Here's how the part is built. I have some questions about the finished solid (model axes, mm). Face numbers are marked on the shaded views. Give positions to 0.01 mm unless a question says otherwise; leave off trailing zeros. Write each loop counter-clockwise with the first axis right and the second up, starting at its lowest first coordinate (ties: lowest second). Pieces come first, ordered by that corner, then holes. Notation, with made-up numbers: (8, 14) - (14, 14) arc R20 cw to (14, 43) - close; hole circle Ø9 at (-6, -35.5). An arc over 180 degrees is marked (long way). One line per item, written item: value. Start each with the question number.
1) I'm going to push flat-ended pins straight in: P1, Ø3.5, axis at x = -12, z = 13, coming from the -Y side; P2, Ø0.9, axis at y = 1.5, z = 2, coming from the +X side; P3, Ø4.5, axis at y = -2, z = 22.5, coming from the -X side; P4, Ø3.5, axis at x = 35.24, y = 12.83, coming from the -Z side. Where does each tip first touch, or does it pass through?
2) Imagine slicing it at A-A on x = 0. Write out the boundary of the cut face in (y, z), plus the area to 3 significant figures.
3) Imagine slicing it at D-D on y = -24. Write out the boundary of the cut face in (x, z).
4) Imagine slicing it at B-B on y = 0. Write out the boundary of the cut face in (x, z), plus the area to 3 significant figures.
5) Imagine slicing it at C-C on z = 8.5. Write out the boundary of the cut face in (x, y).
6) Please list where these lines run through material, in increasing order: L1, parallel to Y at x = 0, z = 22.9; L2, parallel to Z at x = 2.5, y = 6; L3, parallel to Z at x = 24, y = 40. Write a range as [from, to].
7) We'd pull the mould along X, two halves only. Please class the marked faces 1, 2 and 3: +X half, -X half, draft (parallel to the pull), parting line (faces both ways), or undercut.
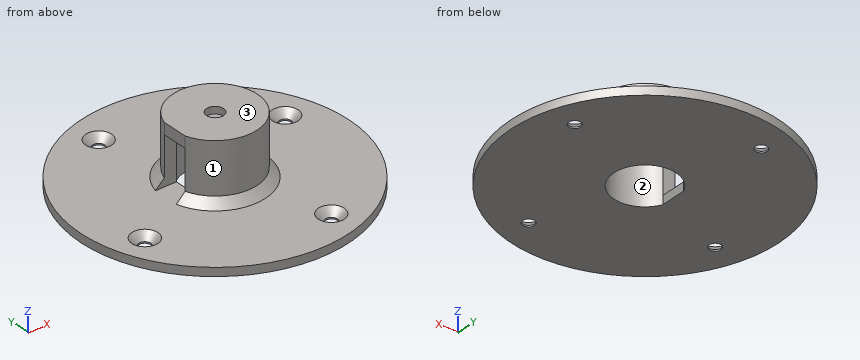
Autodesk Inventor part; units mm, degrees
ref_plane "YZ Plane" through (0, 0, 0) normal (1, 0, 0) x (0, 1, 0)
ref_plane "XZ Plane" through (0, 0, 0) normal (0, 1, 0) x (-1, 0, 0)
ref_plane "XY Plane" through (0, 0, 0) normal (0, 0, 1) x (1, 0, 0)
sketch "Skizze1" plane through (0, 0, 0) normal (0, 0, 1) x (1, 0, 0)
  circle A0 centre (-35.2385, -12.8258) radius 2.1
  circle A1 centre (-12.8258, 35.2385) radius 2.1
  circle A2 centre (12.8258, -35.2385) radius 2.1
  circle A3 centre (35.2385, 12.8258) radius 2.1
  circle A4 centre (0, 0) radius 25
  circle A5 centre (0, 0) radius 45
  circle A6 centre (0, 0) radius 47.5
  circle A7 centre (0, 0) radius 8.4675
  point P0 (0, 0)
extrude "Extrusion1" add sketch "Skizze1" along normal blind 3 contours A4 | A5 | A6 | A7
sketch "Skizze2" plane through (0, 0, 3) normal (0, 0, 1) x (1, 0, 0)
  circle A0 centre (0, 0) radius 15
  dimension "d2" = 30
extrude "Extrusion2" add sketch "Skizze2" along normal blind 21
sketch "Skizze3" plane through (0, 0, 24) normal (0, 0, 1) x (1, 0, 0)
  circle A0 centre (0, 0) radius 3
  dimension "d7" = 6
extrude "Extrusion3" cut sketch "Skizze3" against normal blind 2.5
sketch "Skizze4" plane through (0, 0, 0) normal (0, 0, -1) x (-1, 0, 0)
  circle A0 centre (0, 0) radius 15
  circle A1 centre (0, 0) radius 11
  dimension "d8" = 4
extrude "Extrusion4" cut sketch "Skizze4" against normal blind 20 contours A1
sketch "Skizze5" plane through (0, 0, 0) normal (0, 0, -1) x (-1, 0, 0)
  circle A0 centre (0, 0) radius 11
  circle A1 centre (-35.2385, 12.8258) radius 2.1
  circle A2 centre (-12.8258, -35.2385) radius 2.1
  circle A3 centre (12.8258, 35.2385) radius 2.1
  circle A4 centre (35.2385, -12.8258) radius 2.1
  circle A5 centre (0, 0) radius 47.5
  line L0 (10, -4.5826) -> (10, 4.5826)
  dimension "d11" = 10
extrude "Extrusion5" add sketch "Skizze5" against normal up to surface (20 mm away) contours A0 L0 picked at (10.1839, -1.0361)
sketch "Skizze6" plane through (-10, -4.5826, 0) normal (1, 0, 0) x (0, 0, -1)
  line L0 (-20, 0) -> (-20, 9.1652)
  line L1 (0, 0) -> (-20, 0)
  line L2 (0, 9.1652) -> (0, 0)
  line L3 (-20, 9.1652) -> (0, 9.1652)
  line L4 (-3, -10.4174) -> (-3, 19.5826)
  line L5 (-3, 15.3083) -> (-3, 19.5083)
  line L6 (-3, -32.7559) -> (-3, -28.5559)
  line L7 (-3, 37.721) -> (-3, 41.921)
  line L8 (-3, -10.3432) -> (-3, -6.1432)
  line L9 (-3, 52.0826) -> (-3, -42.9174)
  line L10 (-3, 0) -> (-20, 0)
  line L11 (-20, 0) -> (-20, 9.1652)
  line L12 (-20, 9.1652) -> (-3, 9.1652)
  line L13 (-3, 9.1652) -> (-3, 0)
  point P0 (0, 4.5826)
extrude "Extrusion6" cut sketch "Skizze6" against normal blind 20 contours L0 L3 L4 L1
sketch "Skizze7" plane through (0, 0, 20) normal (0, 0, -1) x (-1, 0, 0)
  arc A0 (10, 4.5826) -> (10, -4.5826) centre (0, 0) ccw
  line L0 (10, -4.5826) -> (14.2829, -4.5826)
  arc A1 (14.2829, -4.5826) -> (14.2829, 4.5826) centre (0, 0) ccw
  line L1 (10, 4.5826) -> (14.2829, 4.5826)
  line L2 (14.2829, 4.5826) -> (14.2829, -4.5826)
extrude "Extrusion7" cut sketch "Skizze7" against normal blind 20 contours A1 L2
chamfer "Fase1" distance 3 angle 45 1 edges at (15, 0, 3)
chamfer "Fase2" distance 2.5 angle 45 4 edges at (-14.9258, 35.2385, 3) (33.1385, 12.8258, 3) (10.7258, -35.2385, 3) (-37.3385, -12.8258, 3)
properties part number "OberArmMagnet" material "ABS-Kunststoff"
Numbers:
1. P1: y = -10.95
1. P2: x = 47.49
1. P3: x = -14.28
1. P4: through
2. outline: (-47.5, 0) - (-11, 0) - (-11, 20) - (11, 20) - (11, 0) - (47.5, 0) - (47.5, 3) - (18, 3) - (15, 6) - (15, 24) - (3, 24) - (3, 21.5) - (-3, 21.5) - (-3, 24) - (-15, 24) - (-15, 6) - (-18, 3) - (-47.5, 3) - close
2. area: 469 mm^2
3. outline: (-40.99, 0) - (40.99, 0) - (40.99, 3) - (-40.99, 3) - close
4. outline: (-47.5, 0) - (-10, 0) - (-10, 3) - (-47.5, 3) - close; (-14.28, 20) - (11, 20) - (11, 0) - (47.5, 0) - (47.5, 3) - (18, 3) - (15, 6) - (15, 24) - (3, 24) - (3, 21.5) - (-3, 21.5) - (-3, 24) - (-14.28, 24) - close
4. area: 397 mm^2
5. outline: (-14.28, -4.58) arc R15 ccw (long way) to (-14.28, 4.58) - (-10, 4.58) arc R11 cw (long way) to (-10, -4.58) - close
6. L1: [-15, -3], [3, 15]
6. L2: [20, 24]
6. L3: [0, 3]
7. face 1: parting line
7. face 2: undercut
7. face 3: draft
